Can you work these out from the model? Positions are in its coordinate system, mm. Face numbers are marked on the shaded views. A direction names the side the tool comes from. Coordinates: 2 decimals unless noted, no trailing zeros. Order: outer loops, then holes, each group sorted by start corner. A loop starts at its lowest first (then second) coordinate and runs counter-clockwise, first axis right, second up. Notation, with made-up numbers: (-4.75, 10) -> (39.25, 10) arc R15 cw to (39.25, 20) -> close; hole circle Ø4 at (16.25, -5). An arc over 180 degrees is marked (long way). Answer in a Markdown table with one row per item.
```python
from build123d import *

# Parameters (mm, degrees)
SKETCH1_W           = 48.26
SKETCH1_H           = 38.1
BOSS_EXTRUDE1_DEPTH = 5.08
SKETCH2_W           = 5.08
SKETCH2_H           = 5.08
CUT_EXTRUDE1_DEPTH  = 5.08


with BuildPart() as part:
    # Sketch1 → Boss-Extrude1 (new body)
    with BuildSketch(Plane(origin=(0, 0, 0), x_dir=(1, 0, 0), z_dir=(0, 1, 0))):
        with Locations((6.327422222, -8.003822222)):
            Rectangle(SKETCH1_W, SKETCH1_H)
    extrude(amount=BOSS_EXTRUDE1_DEPTH)

    # Sketch2 → Cut-Extrude1 (cut)
    with BuildSketch(Plane(origin=(0, 5.08, 0), x_dir=(1, 0, 0), z_dir=(0, 1, 0))):
        with Locations((27.917422222, -24.513822222)):
            Rectangle(SKETCH2_W, SKETCH2_H)
        with Locations((27.917422222, -14.353822222)):
            Rectangle(SKETCH2_W, SKETCH2_H)
        with Locations((-15.262577778, 8.506177778)):
            Rectangle(SKETCH2_W, SKETCH2_H)
        with Locations((-15.262577778, -1.653822222)):
            Rectangle(SKETCH2_W, SKETCH2_H)
        with Locations((-15.262577778, -24.513822222)):
            Rectangle(SKETCH2_W, SKETCH2_H)
        with Locations((-15.262577778, -14.353822222)):
            Rectangle(SKETCH2_W, SKETCH2_H)
        with Locations((27.917422222, -1.653822222)):
            Rectangle(SKETCH2_W, SKETCH2_H)
        with Locations((27.917422222, 8.506177778)):
            Rectangle(SKETCH2_W, SKETCH2_H)
    extrude(amount=-CUT_EXTRUDE1_DEPTH, mode=Mode.SUBTRACT)


solid = part.part
```
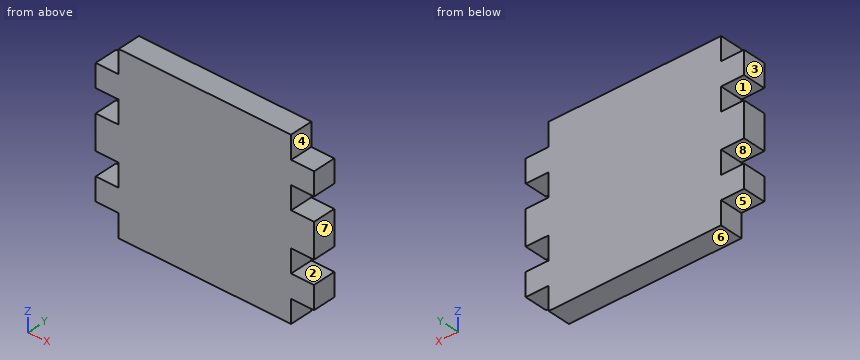
(1) Suppose I cut it at B-B (y = 1). Please give me the cut outline in (x, z), and give its area (3 significant figures).
Response values:
| item | result |
|---|---|
| outline | (-17.8, -5.97) -> (-12.72, -5.97) -> (-12.72, -11.05) -> (25.38, -11.05) -> (25.38, -5.97) -> (30.46, -5.97) -> (30.46, -0.89) -> (25.38, -0.89) -> (25.38, 4.19) -> (30.46, 4.19) -> (30.46, 11.81) -> (25.38, 11.81) -> (25.38, 16.89) -> (30.46, 16.89) -> (30.46, 21.97) -> (25.38, 21.97) -> (25.38, 27.05) -> (-12.72, 27.05) -> (-12.72, 21.97) -> (-17.8, 21.97) -> (-17.8, 16.89) -> (-12.72, 16.89) -> (-12.72, 11.81) -> (-17.8, 11.81) -> (-17.8, 4.19) -> (-12.72, 4.19) -> (-12.72, -0.89) -> (-17.8, -0.89) -> close |
| area | 1,630 mm2 |
(2) Suppose I cut it at A-A (x = 26). Please give me the cut outline in (y, z).
Response values:
| item | result |
|---|---|
| outline | (0, -5.97) -> (5.08, -5.97) -> (5.08, -0.89) -> (0, -0.89) -> close; (0, 4.19) -> (5.08, 4.19) -> (5.08, 11.81) -> (0, 11.81) -> close; (0, 16.89) -> (5.08, 16.89) -> (5.08, 21.97) -> (0, 21.97) -> close |
(3) We'd pull the mould along Z, two halves only. Please class the marked faces 6, 7 and 8: +Z half, -Z half, draft (parallel to the pull), parting line (faces both ways), or undercut.
Response values:
| item | result |
|---|---|
| face 6 | -Z half |
| face 7 | draft |
| face 8 | undercut |
(4) Suppose I cut it at C-C (z = 12.5). Please give me the cut outline in (x, y), and give its area (3 significant figures).
Response values:
| item | result |
|---|---|
| outline | (-12.72, 0) -> (25.38, 0) -> (25.38, 5.08) -> (-12.72, 5.08) -> close |
| area | 194 mm2 |
(5) On a 3-axis mill with a long thin cutter (end or side, diameter ignored), from which of +Z, -Z, +X, -X, +Y, -Y can I reach the whole of each face in a straight line? I mean the marked faces 1, 2, 3, 4 and 5. Say none if no direction works.
Response values:
| item | result |
|---|---|
| face 1 | -X, +Y, -Y |
| face 2 | +X, +Y, -Y |
| face 3 | +Z, -Z, -X, +Y, -Y |
| face 4 | +Z, +X, +Y, -Y |
| face 5 | -Z, -X, +Y, -Y |
(6) I need wall thicknesses on line 1 (Z direction, x = 27.5, y = 0.3); line 2 (X direction, y = 0.65, z = 2). Which ranges of each line are inside material? Lowest first, please. Write a range as [from, to].
Response values:
| item | result |
|---|---|
| line 1 | [-5.97, -0.89], [4.19, 11.81], [16.89, 21.97] |
| line 2 | [-12.72, 25.38] |
(7) Will these pins go through, and if not, where does the flat tip stop? pin 1 Ø1 at (y, z) = (1, -6.5) entering from +X; pin 2 Ø2.5 at (x, y) = (27, 1.5) entering from +Z; pin 3 Ø2 at (x, z) = (-1.5, -6) entering from -Y; pin 4 Ø2.5 at (y, z) = (2.5, -7.5) entering from -X.
Response values:
| item | result |
|---|---|
| pin 1 | x = 25.38 |
| pin 2 | z = 21.97 |
| pin 3 | y = 0 |
| pin 4 | x = -12.72 |
